Can you work these out from the model? Positions are in its coordinate system, mm. Round coordinates to 2 decimals unless told otherwise and drop trailing zeros. Loops run counter-clockwise (first coordinate to the right, second up) from the corner with the lowest first, then second, coordinate; pieces in that order, holes last. Notation, with made-up numbers: M 48,-29 L 94,-29 A28 cw 94,6 Z; hole C 35.25,-29.75 d5. An arc over 180 degrees is marked long. Use a Markdown table: item, result. Add a question column.
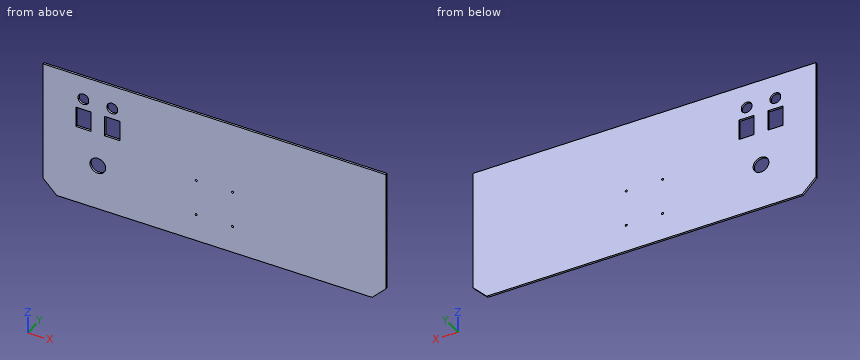
```python
from build123d import *

# Parameters (mm, degrees)
BOSS_EXTRUDE1_DEPTH = 3
SKETCH2_R           = 1.5
CUT_EXTRUDE1_DEPTH  = 3
SKETCH3_R           = 11.5
SKETCH3_W           = 22
SKETCH3_H           = 30
CUT_EXTRUDE2_DEPTH  = 3
CUT_EXTRUDE3_DEPTH  = 3


with BuildPart() as part:
    # Sketch1 → Boss-Extrude1 (new body)
    with BuildSketch(Plane(origin=(0, 0, 0), x_dir=(1, 0, 0), z_dir=(0, 1, 0))):
        Polygon((219.069498766, 78.55), (219.069498766, -98.55), (-280.930501234, -98.55), (-280.930501234, 78.55), (-260.930501234, 98.55), (199.069498766, 98.55), align=None)
    extrude(amount=BOSS_EXTRUDE1_DEPTH)

    # Sketch2 → Cut-Extrude1 (cut)
    with BuildSketch(Plane(origin=(0, 3, 0), x_dir=(1, 0, 0), z_dir=(0, 1, 0))):
        with Locations((-4.430501234, 5.55)):
            Circle(SKETCH2_R)
        with Locations((-57.430501234, 5.55)):
            Circle(SKETCH2_R)
        with Locations((-57.430501234, 58.55)):
            Circle(SKETCH2_R)
        with Locations((-4.430501234, 58.55)):
            Circle(SKETCH2_R)
    extrude(amount=-CUT_EXTRUDE1_DEPTH, mode=Mode.SUBTRACT)

    # Sketch3 → Cut-Extrude2 (cut)
    with BuildSketch(Plane(origin=(0, 3, 0), x_dir=(1, 0, 0), z_dir=(0, 1, 0))):
        with Locations((-200.930501234, 32.05)):
            Circle(SKETCH3_R)
        with Locations((-221.930501234, -32.95)):
            Rectangle(SKETCH3_W, SKETCH3_H)
        with Locations((-179.930501234, -32.95)):
            Rectangle(SKETCH3_W, SKETCH3_H)
    extrude(amount=-CUT_EXTRUDE2_DEPTH, mode=Mode.SUBTRACT)

    # Sketch4 → Cut-Extrude3 (cut)
    with BuildSketch(Plane(origin=(0, 3, 0), x_dir=(1, 0, 0), z_dir=(0, 1, 0))):
        with BuildLine():
            Line((-187.630501234, -61.779746559), (-187.630501234, -66.120253441))
            ThreePointArc((-187.630501234, -66.120253441), (-179.930501234, -71.95), (-172.230501234, -66.120253441))
            Line((-172.230501234, -66.120253441), (-172.230501234, -61.779746559))
            ThreePointArc((-172.230501234, -61.779746559), (-179.930501234, -55.95), (-187.630501234, -61.779746559))
        make_face()
        with BuildLine():
            Line((-229.630501234, -61.779746559), (-229.630501234, -66.120253441))
            ThreePointArc((-229.630501234, -66.120253441), (-221.930501234, -71.95), (-214.230501234, -66.120253441))
            Line((-214.230501234, -66.120253441), (-214.230501234, -61.779746559))
            ThreePointArc((-214.230501234, -61.779746559), (-221.930501234, -55.95), (-229.630501234, -61.779746559))
        make_face()
    extrude(amount=-CUT_EXTRUDE3_DEPTH, mode=Mode.SUBTRACT)


solid = part.part
```
(1) If I drill on probe 1 along X at (y, z) = (1.6, -58.55); probe 2 along X at (y, z) = (1.2, 33); probe 3 along X at (y, z) = (0.65, -33), over which ranges is the centre line in solid material (lowest first)? Write a range as [from, to].
(2) Suppose I cut it at B-B on y = 1.55. Count the separate pieces of the cut face and the enclosed holes in it, and give its area (3 significant figures).
(3) Suppose I cut it at A-A on z = -32.05. List the corners of the cut face in (x, y) for me.
(4) I'm going to push a flat-ended pin straight in: pin 1 (20.5 mm diameter, centred on x = -200.93, z = -32.05, fed in from -Y). Where does the tip first touch, or does it pass through?
Results below:
| question | item | result |
|---|---|---|
| 1 | probe 1 | x = [-280.93, -58.93], [-55.93, -5.93], [-2.93, 219.07] |
| 1 | probe 2 | x = [-280.93, -232.93], [-210.93, -190.93], [-168.93, 219.07] |
| 1 | probe 3 | x = [-280.93, -212.39], [-189.47, 219.07] |
| 2 | separate pieces | 1 |
| 2 | enclosed holes | 9 |
| 2 | area | 96,000 mm² |
| 3 | outline | M -280.93,0 L -212.43,0 L -212.43,3 L -280.93,3 Z; M -189.43,0 L 219.07,0 L 219.07,3 L -189.43,3 Z |
| 4 | pin 1 | passes through |
